```python
from build123d import *

# Parameters (mm, degrees)
BOSS_EXTRUDE1_DEPTH = 10
SKETCH5_R           = 4
CUT_EXTRUDE3_DEPTH  = 5
CUT_EXTRUDE1_REACH  = 52.252
SKETCH3_R           = 1.65
CUT_EXTRUDE2_DEPTH  = 3.3
FILLET1_R           = 1.65


with BuildPart() as part:
    # Sketch1 → Boss-Extrude1 (new body)
    with BuildSketch(Plane.XY):
        with BuildLine():
            Line((-10, -47.5), (10, -47.5))
            ThreePointArc((10, -47.5), (12.121320344, -46.621320344), (13, -44.5))
            Line((13, -44.5), (13, 4.5))
            ThreePointArc((13, 4.5), (12.121320344, 6.621320344), (10, 7.5))
            Line((10, 7.5), (-10, 7.5))
            ThreePointArc((-10, 7.5), (-12.121320344, 6.621320344), (-13, 4.5))
            Line((-13, 4.5), (-13, -44.5))
            ThreePointArc((-13, -44.5), (-12.121320344, -46.621320344), (-10, -47.5))
        make_face()
    extrude(amount=BOSS_EXTRUDE1_DEPTH)

    # Sketch5 → Cut-Extrude3 (cut)
    with BuildSketch(Plane(origin=(0, 0, 0), x_dir=(-1, 0, 0), z_dir=(0, 0, -1))):
        with Locations((0, -20)):
            Circle(SKETCH5_R)
    extrude(amount=-CUT_EXTRUDE3_DEPTH, mode=Mode.SUBTRACT)

    # Cut-Extrude1: up to this face of the body (flat: up to its plane)
    cut_extrude1_end = Plane(part.part.faces().sort_by_distance((-11.69114596, -46.19114596, 0))[0])
    # Sketch2 → Cut-Extrude1 (cut, up to the picked face)
    with BuildSketch(Plane.XY.offset(10), mode=Mode.PRIVATE) as cut_extrude1_sk1:
        with BuildLine():
            Line((-1.322875656, -18.5), (-7.858116823, -18.5))
            Line((-7.858116823, -18.5), (-7.858116823, -21.5))
            Line((-7.858116823, -21.5), (-1.322875656, -21.5))
            ThreePointArc((-1.322875656, -21.5), (2, -20), (-1.322875656, -18.5))
        make_face()
    cut_extrude1_tool1 = split(extrude(cut_extrude1_sk1.sketch, amount=-CUT_EXTRUDE1_REACH, mode=Mode.PRIVATE), bisect_by=cut_extrude1_end, keep=Keep.BOTH, mode=Mode.PRIVATE)
    add(cut_extrude1_tool1.solids().sort_by(Axis((-2.852345, -20, 10), (0, 0, -1)))[0], mode=Mode.SUBTRACT)

    # Sketch3 → Cut-Extrude2 (cut)
    with BuildSketch(Plane(origin=(0, 0, 0), x_dir=(-1, 0, 0), z_dir=(0, 0, -1))):
        with Locations((0, -5.5)):
            Circle(SKETCH3_R)
        with Locations((0, -9)):
            Circle(SKETCH3_R)
        with Locations((0, -12.5)):
            Circle(SKETCH3_R)
    extrude(amount=-CUT_EXTRUDE2_DEPTH, mode=Mode.SUBTRACT)

    # Fillet1
    fillet1_edges = [part.edges().sort_by_distance(p)[0] for p in [
        (1.65, -5.5, 3.3),
        (1.65, -9, 3.3),
        (1.65, -12.5, 3.3),
    ]]
    fillet(fillet1_edges, radius=FILLET1_R)


solid = part.part
```
Read the model definition and answer for the solid it produces. Units are mm, in the model's axes. A direction names the side the tool comes from. Round coordinates to 2 decimals unless told otherwise and drop trailing zeros. Write each loop counter-clockwise with the first axis right and the second up, starting at its lowest first coordinate (ties: lowest second). Pieces come first, ordered by that corner, then holes. Notation, with made-up numbers: (78, 89) - (101, 89) arc R21 cw to (101, 126) - close; hole circle Ø3 at (-38.75, 5). An arc over 180 degrees is marked (long way). One line per item, written item: value.
Q1. Find section A-A (x = 0). Determine the outline of the cut face in (y, z), and give its area (3 significant figures).
The answers:
outline: (-47.5, 0) - (-24, 0) - (-24, 5) - (-22, 5) - (-22, 10) - (-47.5, 10) - close; (-18, 5) - (-16, 5) - (-16, 0) - (-14.15, 0) - (-14.15, 1.65) arc R1.65 cw to (-10.85, 1.65) - (-10.85, 0) - (-10.65, 0) - (-10.65, 1.65) arc R1.65 cw to (-7.35, 1.65) - (-7.35, 0) - (-7.15, 0) - (-7.15, 1.65) arc R1.65 cw to (-3.85, 1.65) - (-3.85, 0) - (7.5, 0) - (7.5, 10) - (-18, 10) - close
area: 461 mm2
Q2. Each of these flat-tipped pins is pushed along its axis until it touches: P1, Ø2, axis at x = 0, y = -12.5, coming from the -Z side; P2, Ø5, axis at x = 0, y = -20, coming from the -Z side. Where does it stop, or does it pass through?
The answers:
P1: stops at z = 2.96
P2: stops at z = 5
Q3. Find section C-C (y = -20). Determine the outline of the cut face in (x, z), and give its area (3 significant figures).
The answers:
outline: (-13, 0) - (-7.86, 0) - (-7.86, 10) - (-13, 10) - close; (2, 5) - (4, 5) - (4, 0) - (13, 0) - (13, 10) - (2, 10) - close
area: 151 mm2
Q4. Find section D-D (y = -12.5). Determine the outline of the cut face in (x, z).
The answers:
outline: (-13, 0) - (-1.65, 0) - (-1.65, 1.65) arc R1.65 cw to (1.65, 1.65) - (1.65, 0) - (13, 0) - (13, 10) - (-13, 10) - close
Q5. Find section B-B (z = 4). Determine the outline of the cut face in (x, y).
The answers:
outline: (-13, -44.5) arc R3 ccw to (-10, -47.5) - (10, -47.5) arc R3 ccw to (13, -44.5) - (13, 4.5) arc R3 ccw to (10, 7.5) - (-10, 7.5) arc R3 ccw to (-13, 4.5) - close; hole (-7.86, -21.5) - (-3.71, -21.5) arc R4 ccw (long way) to (-3.71, -18.5) - (-7.86, -18.5) - close
Q6. For a pull along Y with two mould halves and no side action, classify faces 1 (the flat face through (13, -20, 5)), 2 (the cylindrical face through (12.1, -46.64, 4.93)), 3 (the cylindrical face through (2, -20, 8)) as pulls with the +Y half, pulls with the -Y half, needs draft (parallel to the pull), parting line crosses it, or undercut.
The answers:
face 1: needs draft
face 2: pulls with the -Y half
face 3: undercut
Q7. Which of the six approach directions +Z, -Z, +X, -X, +Y, -Y give full straight-line access (tool end or side, diameter ignored) to faces 4 (the cylindrical face through (1.31, -10, 0.81)), 5 (the flat face through (-5, -21.5, 5)), 6 (the cylindrical face through (-12.1, 6.64, 4.93))?
The answers:
face 4: -Z
face 5: +Z, -Z
face 6: +Z, -Z, -X, +Y
Q8. Straight lines are drawn through the part: line 1 (Y direction, x = 0, z = 0.75); line 2 (Y direction, x = 0, z = 8.05); line 3 (Y direction, x = 0.75, z = 1.25). For each, find the intervals that lie inside material, in ascending order. Write a range as from..to.
The answers:
line 1: y = -47.5..-24, -16..-14.15, -10.85..-10.65, -7.35..-7.15, -3.85..7.5
line 2: y = -47.5..-22, -18..7.5
line 3: y = -47.5..-23.93, -16.07..-13.97, -11.03..-10.47, -7.53..-6.97, -4.03..7.5
